```python
from build123d import *

# Parameters (mm, degrees)
SKETCH1_R                                           = 75
BOSS_EXTRUDE1_DEPTH                                 = 5
CSK_FOR_M3_COUNTERSUNK_FLAT_HEAD_SCREW1_D           = 3.4
CSK_FOR_M3_COUNTERSUNK_FLAT_HEAD_SCREW1_CSINK_D     = 6.3
CSK_FOR_M3_COUNTERSUNK_FLAT_HEAD_SCREW1_CSINK_ANGLE = 90
SKETCH5_R                                           = 7.5
CUT_EXTRUDE1_DEPTH                                  = 107.183802908


with BuildPart() as part:
    # Sketch1 → Boss-Extrude1 (new body)
    with BuildSketch(Plane(origin=(0, 0, 0), x_dir=(1, 0, 0), z_dir=(0, 1, 0))):
        with Locations(Location((0, 0, 0), (0, 0, 270))):
            Circle(SKETCH1_R)
    extrude(amount=BOSS_EXTRUDE1_DEPTH)

    # CSK for M3 Countersunk Flat Head Screw1 (through all)
    with Locations(Plane(origin=(0, 5, 0), x_dir=(1, 0, 0), z_dir=(0, 1, 0))):
        with Locations((-40, 40), (40, 40), (40, -40), (-40, -40)):
            CounterSinkHole(CSK_FOR_M3_COUNTERSUNK_FLAT_HEAD_SCREW1_D / 2, CSK_FOR_M3_COUNTERSUNK_FLAT_HEAD_SCREW1_CSINK_D / 2, counter_sink_angle=CSK_FOR_M3_COUNTERSUNK_FLAT_HEAD_SCREW1_CSINK_ANGLE)

    # Sketch5 → Cut-Extrude1 (cut, through all)
    with BuildSketch(Plane(origin=(0, 5, 0), x_dir=(1, 0, 0), z_dir=(0, 1, 0))):
        with Locations(Location((0, 0, 0), (0, 0, 270))):
            Circle(SKETCH5_R)
    extrude(amount=-CUT_EXTRUDE1_DEPTH, mode=Mode.SUBTRACT)


solid = part.part
```
Read the model definition and answer for the solid it produces. Units are mm, in the model's axes. Give positions to 0.01 mm unless a question says otherwise; leave off trailing zeros. Write each loop counter-clockwise with the first axis right and the second up, starting at its lowest first coordinate (ties: lowest second). Pieces come first, ordered by that corner, then holes. Notation, with made-up numbers: M 30,40 L 82,40 A35 ccw 82,75 Z; hole C 70,34.5 d3. An arc over 180 degrees is marked long. Put each result on its own line as item: value. Start each with the question number.
1. For a pull along Z with two mould halves and no side action, classify faces 1 (the flat face through (-16, 5, -1)), 2 (the cylindrical face through (-38.65, 1.75, 41.03)), 3 (the cylindrical face through (-45.636, 2.465, -59.517)) as released by +Z, released by -Z, zero draft, split by the parting line, or undercut.
2. The part is cut by section B-B, the plane z = 0. Give the vertices of the cut face in (x, y).
3. Consider line 1 along Z through (x, y) = (40, 2.6); line 2 along Z through (x, y) = (-40.5, 3.5). Determine where each line is inside the solid, lowest interval first.
4. The part is cut by section C-C, the plane y = 1. Give the vertices of the cut face in (x, z).
5. Each of these flat-tipped pins is pushed along its axis until it touches: pin 1 Ø13.5 at (x, z) = (0, 0) entering from +Y; pin 2 Ø3 at (y, z) = (1.5, -41) entering from -X; pin 3 Ø3 at (x, y) = (43.5, 2.5) entering from -Z; pin 4 Ø3 at (y, z) = (2, 35.5) entering from -X. Where does it stop, or does it pass through?
6. The part is cut by section D-D, the plane x = 40. Give the vertices of the cut face in (y, z), and give its area (3 significant figures).
7. The part is cut by section A-A, the plane x = 0. Give the vertices of the cut face in (y, z), and give its area (3 significant figures).
Final values:
1. face 1: zero draft
1. face 2: undercut
1. face 3: split by the parting line
2. outline: M -75,0 L -7.5,0 L -7.5,5 L -75,5 Z; M 7.5,0 L 75,0 L 75,5 L 7.5,5 Z
3. line 1: z = -63.44 to -41.7, -38.3 to 38.3, 41.7 to 63.44
3. line 2: z = -63.12 to -41.62, -38.38 to 38.38, 41.62 to 63.12
4. outline: C 0,0 d150; hole C -40,-40 d3.4; hole C -40,40 d3.4; hole C 0,0 d15; hole C 40,-40 d3.4; hole C 40,40 d3.4
5. pin 1: passes through
5. pin 2: stops at x = -63.76
5. pin 3: stops at z = -62.14
5. pin 4: stops at x = -66.85
6. outline: M 0,-63.44 L 5,-63.44 L 5,-43.15 L 3.55,-41.7 L 0,-41.7 Z; M 0,-38.3 L 3.55,-38.3 L 5,-36.85 L 5,36.85 L 3.55,38.3 L 0,38.3 Z; M 0,41.7 L 3.55,41.7 L 5,43.15 L 5,63.44 L 0,63.44 Z
6. area: 596 mm²
7. outline: M 0,-75 L 5,-75 L 5,-7.5 L 0,-7.5 Z; M 0,7.5 L 5,7.5 L 5,75 L 0,75 Z
7. area: 675 mm²
